from build123d import *

# Parameters (mm, degrees)
ESQUISSE1_W             = 43
ESQUISSE1_H             = 20
BOSS_EXTRU_1_DEPTH      = 52
ESQUISSE2_W             = 57.277645312
ESQUISSE2_H             = 21.944309951
ENL_V_MAT_EXTRU_1_DEPTH = 50
D_GAGEMENT_M41_D        = 4.5
D_GAGEMENT_M51_D        = 5.5


with BuildPart() as part:
    # Esquisse1 → Boss.-Extru.1 (new body)
    with BuildSketch(Plane.XY):
        Rectangle(ESQUISSE1_W, ESQUISSE1_H)
    extrude(amount=BOSS_EXTRU_1_DEPTH)

    # Esquisse2 → Enlèv. mat.-Extru.1 (cut)
    with BuildSketch(Plane.XY.offset(52)):
        with Locations((1.570038745, -2.972154976)):
            Rectangle(ESQUISSE2_W, ESQUISSE2_H)
    extrude(amount=-ENL_V_MAT_EXTRU_1_DEPTH, mode=Mode.SUBTRACT)

    # Dégagement M41 (through all)
    with Locations(Plane(origin=(0, 10, 0), x_dir=(1, 0, 0), z_dir=(0, 1, 0))):
        with Locations((-0.5, -21.95), (-0.5, -32.95), (-0.5, -43.95), (-8.5, -32.95)):
            Hole(D_GAGEMENT_M41_D / 2)

    # Dégagement M51 (through all)
    with Locations(Plane(origin=(0, 0, 0), x_dir=(-1, 0, 0), z_dir=(0, 0, -1))):
        with Locations((-11.632687115, 0), (8.686603755, 0)):
            Hole(D_GAGEMENT_M51_D / 2)


solid = part.part
The listing builds one solid part. Answer for the finished solid, in the listing's coordinates (mm). A direction names the side the tool comes from. Round coordinates to 2 decimals unless told otherwise and drop trailing zeros. Order: outer loops, then holes, each group sorted by start corner. A loop starts at its lowest first (then second) coordinate and runs counter-clockwise, first axis right, second up. Notation, with made-up numbers: (-6, -6.5) - (12, -6.5) arc R9 ccw to (12, 3.5) - close; hole circle Ø5 at (-13, -23.5). An arc over 180 degrees is marked (long way). Write item = value, one per line. Start each with the question number.
1) Section C-C, the plane z = 21.95 is taken. Write down the section's boundary in (x, y).
2) Given pin 1 (4 mm diameter, centred on x = -0.5, z = 32.95, fed in from -Y); pin 2 (9 mm diameter, centred on x = 2.5, y = 2.5, fed in from +Z); pin 3 (13 mm diameter, centred on x = 5, z = 36, fed in from -Y), each flat-ended and moving along its own axis, determine where each tip first touches the part or whether it passes through.
3) Straight lines are drawn through the part: L1, parallel to X at y = 8.5, z = 32.95; L2, parallel to X at y = 8.9, z = 21.95; L3, parallel to Y at x = -18, z = 8. For each, find the intervals that lie inside material, in ascending order.
4) Section D-D, the plane x = -8.5 is taken. Write down the section's boundary in (y, z), plus the area to 3 significant figures.
5) For a pull along Z with two mould halves and no side action, classify faces 3 (the flat face through (0, -10, 1)), 4 (the flat face through (0, -1, 2)), 5 (the cylindrical face through (-0.012, 8.986, 24.146)) as released by +Z, released by -Z, zero draft, split by the parting line, or undercut.
6) Section A-A, the plane x = -0.5 is taken. Write down the section's boundary in (y, z), plus the area to 3 significant figures.
7) For faces 1 (the flat face through (0, 8, 27)), 2 (the cylindrical face through (-0.012, 8.986, 46.146)), determine the directions among +Z, -Z, +X, -X, +Y, -Y from which every point of the face is accessible in a straight line to the end or side of a thin tool.
8) Section B-B, the plane z = 32.95 is taken. Write down the section's boundary in (x, y), plus the area to 3 significant figures.
Results list:
q1.outline = (-21.5, 8) - (-2.75, 8) - (-2.75, 10) - (-21.5, 10) - close; (1.75, 8) - (21.5, 8) - (21.5, 10) - (1.75, 10) - close
q2.pin_1 = through
q2.pin_2 = 2
q2.pin_3 = 8
q3.L1 = -21.5 to -10.75, -6.25 to -2.75, 1.75 to 21.5
q3.L2 = -21.5 to -2.75, 1.75 to 21.5
q3.L3 = 8 to 10
q4.outline = (-10, 0) - (-2.74, 0) - (-2.74, 2) - (-10, 2) - close; (2.74, 0) - (10, 0) - (10, 30.7) - (8, 30.7) - (8, 2) - (2.74, 2) - close; (8, 35.2) - (10, 35.2) - (10, 52) - (8, 52) - close
q4.area = 120 mm^2
q5.face_3 = zero draft
q5.face_4 = released by +Z
q5.face_5 = undercut
q6.outline = (-10, 0) - (10, 0) - (10, 19.7) - (8, 19.7) - (8, 2) - (-10, 2) - close; (8, 24.2) - (10, 24.2) - (10, 30.7) - (8, 30.7) - close; (8, 35.2) - (10, 35.2) - (10, 41.7) - (8, 41.7) - close; (8, 46.2) - (10, 46.2) - (10, 52) - (8, 52) - close
q6.area = 113 mm^2
q7.face_1 = +Z, +X, -X, -Y
q7.face_2 = +Y, -Y
q8.outline = (-21.5, 8) - (-10.75, 8) - (-10.75, 10) - (-21.5, 10) - close; (-6.25, 8) - (-2.75, 8) - (-2.75, 10) - (-6.25, 10) - close; (1.75, 8) - (21.5, 8) - (21.5, 10) - (1.75, 10) - close
q8.area = 68.0 mm^2
